Build history of the part. All positions in model axes, mm. Face numbers are marked on the shaded views. A direction names the side the tool comes from. Round coordinates to 2 decimals unless told otherwise and drop trailing zeros. Loops run counter-clockwise (first coordinate to the right, second up) from the corner with the lowest first, then second, coordinate; pieces in that order, holes last.
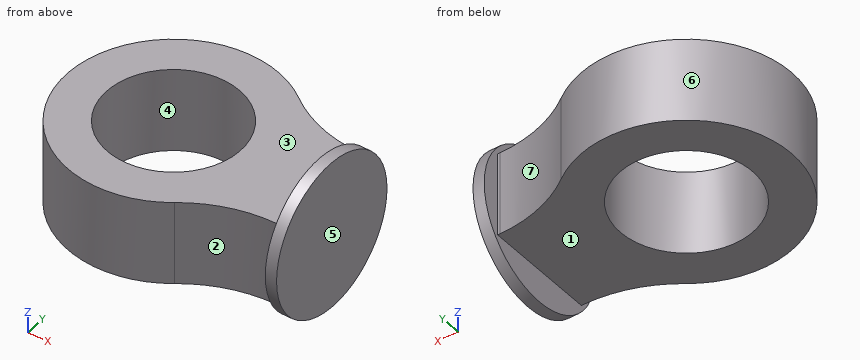
from build123d import *

# Parameters (mm, degrees)
SKETCH1_R           = 29.25
BOSS_EXTRUDE1_DEPTH = 37
SKETCH2_R           = 33
BOSS_EXTRUDE2_DEPTH = 5


with BuildPart() as part:
    # Sketch1 → Boss-Extrude1 (new body)
    with BuildSketch(Plane.XY):
        with BuildLine():
            Line((64.16580086, 25), (65.20777984, 25))
            Line((65.20777984, 25), (65.20777984, -25))
            Line((65.20777984, -25), (64.16580086, -25))
            ThreePointArc((64.16580086, -25), (45.103264783, -28.108702614), (28.016053897, -37.112676056))
            ThreePointArc((28.016053897, -37.112676056), (-46.5, 0), (28.016053897, 37.112676056))
            ThreePointArc((28.016053897, 37.112676056), (45.103264783, 28.108702614), (64.16580086, 25))
        make_face()
        Circle(SKETCH1_R, mode=Mode.SUBTRACT)
    extrude(amount=BOSS_EXTRUDE1_DEPTH)

    # Sketch2 → Boss-Extrude2 (add)
    with BuildSketch(Plane(origin=(65.20777984, 0, 0), x_dir=(0, 0, -1), z_dir=(1, 0, 0))):
        with Locations((-18.5, 0)):
            Circle(SKETCH2_R)
    extrude(amount=BOSS_EXTRUDE2_DEPTH)


solid = part.part
(1) Slice it at A-A on x = 0. List the corners of the cut face in (y, z), plus the area to 3 significant figures.
Responses:
outline: (-46.5, 0) - (-29.25, 0) - (-29.25, 37) - (-46.5, 37) - close; (29.25, 0) - (46.5, 0) - (46.5, 37) - (29.25, 37) - close
area: 1,280 mm2
(2) Slice it at B-B on y = -15.5. List the corners of the cut face in (x, z), plus the area to 3 significant figures.
Responses:
outline: (-43.84, 0) - (-24.81, 0) - (-24.81, 37) - (-43.84, 37) - close; (24.81, 0) - (65.21, 0) - (65.21, -10.63) - (70.21, -10.63) - (70.21, 47.63) - (65.21, 47.63) - (65.21, 37) - (24.81, 37) - close
area: 2,490 mm2
(3) Probe line 1 (Z direction, x = 52.5, y = 13.5); line 2 (Y direction, x = -18.5, z = 14); line 3 (X direction, y = -5.5, z = 41.5). List the from-to ranges inside material, lowest first.
Responses:
line 1: z = 0 to 37
line 2: y = -42.66 to -22.66, 22.66 to 42.66
line 3: x = 65.21 to 70.21
(4) Slice it at D-D on y = 6. List the corners of the cut face in (x, z), plus the area to 3 significant figures.
Responses:
outline: (-46.11, 0) - (-28.63, 0) - (-28.63, 37) - (-46.11, 37) - close; (28.63, 0) - (65.21, 0) - (65.21, -13.95) - (70.21, -13.95) - (70.21, 50.95) - (65.21, 50.95) - (65.21, 37) - (28.63, 37) - close
area: 2,320 mm2
(5) Which spindle directions (+Z, -Z, +X, -X, +Y, -Y) get a long thin tool onto all of the face, cutting with end or side? Do the marked faces 1, 2 and 3. Say none if no direction does.
Responses:
face 1: -Z, -X, +Y, -Y
face 2: +Z, -Z, -Y
face 3: +Z, -X, +Y, -Y
(6) Slice it at C-C on z = 24. List the corners of the cut face in (x, y), plus the area to 3 significant figures.
Responses:
outline: (28.02, -37.11) arc R60 cw to (64.17, -25) - (65.21, -25) - (65.21, -32.54) - (70.21, -32.54) - (70.21, 32.54) - (65.21, 32.54) - (65.21, 25) - (64.17, 25) arc R60 cw to (28.02, 37.11) arc R46.5 ccw (long way) to start; hole circle Ø58.5 at (0, 0)
area: 5,610 mm2
(7) Pin check, flat tips, straight feed: P1, Ø3, axis at y = 17.5, z = 22, coming from the -X side; P2, Ø5, axis at x = 47.5, y = -8, coming from the -Z side; P3, Ø1.1, axis at x = 64.5, z = 11.5, coming from the -Y side. Stop position of each tip, or through.
Responses:
P1: stops at x = -43.66
P2: stops at z = 0
P3: stops at y = -25
(8) Pull direction X, two halves, no side cores. Call the marked faces 4, 5, 6 and 7: +X half, -X half, draft (parallel to the pull), parting line (faces both ways), or undercut.
Responses:
face 4: undercut
face 5: +X half
face 6: parting line
face 7: undercut
